Read the model definition and answer for the solid it produces. Units are mm, in the model's axes. A direction names the side the tool comes from. Coordinates: 2 decimals unless noted, no trailing zeros. Order: outer loops, then holes, each group sorted by start corner. A loop starts at its lowest first (then second) coordinate and runs counter-clockwise, first axis right, second up. Notation, with made-up numbers: (11.25, -29.5) -> (50.25, -29.5) arc R17 cw to (50.25, -22.5) -> close; hole circle Ø2 at (32, 68). An arc over 180 degrees is marked (long way). Answer in a Markdown table with one row per item.
from build123d import *

# Parameters (mm, degrees)
SKETCH1_W           = 35
SKETCH1_H           = 40
BOSS_EXTRUDE1_DEPTH = 2
SKETCH2_R           = 2.5
CUT_EXTRUDE1_DEPTH  = 54.188344588
SKETCH3_R           = 5.071067812
BOSS_EXTRUDE2_DEPTH = 35


with BuildPart() as part:
    # Sketch1 → Boss-Extrude1 (new body)
    with BuildSketch(Plane.XY):
        with Locations((17.5, 20)):
            Rectangle(SKETCH1_W, SKETCH1_H)
    extrude(amount=BOSS_EXTRUDE1_DEPTH)

    # Sketch2 → Cut-Extrude1 (cut, through all)
    with BuildSketch(Plane(origin=(0, 0, 0), x_dir=(-1, 0, 0), z_dir=(0, 0, -1))):
        with Locations((-27, 24)):
            Circle(SKETCH2_R)
        with Locations((-8, 24)):
            Circle(SKETCH2_R)
        with Locations((-8, 7.5)):
            Circle(SKETCH2_R)
        with Locations((-27, 7.5)):
            Circle(SKETCH2_R)
    extrude(amount=-CUT_EXTRUDE1_DEPTH, mode=Mode.SUBTRACT)

    # Sketch3 → Boss-Extrude2 (add)
    with BuildSketch(Plane.ZY):
        with BuildLine():
            Line((0, 40), (2, 40))
            Line((2, 40), (2, 44))
            ThreePointArc((2, 44), (1, 58.071067812), (0, 44))
            Line((0, 44), (0, 40))
        make_face()
        with Locations((1, 51)):
            Circle(SKETCH3_R, mode=Mode.SUBTRACT)
    extrude(amount=-BOSS_EXTRUDE2_DEPTH)


solid = part.part
Q1. The part is cut by section A-A (z = 1). Write down the section's boundary in (x, y).
Outcome:
| item | result |
|---|---|
| outline | (0, 0) -> (35, 0) -> (35, 45.93) -> (0, 45.93) -> close; (0, 56.07) -> (35, 56.07) -> (35, 58.07) -> (0, 58.07) -> close; hole circle Ø5 at (8, 7.5); hole circle Ø5 at (8, 24); hole circle Ø5 at (27, 7.5); hole circle Ø5 at (27, 24) |
Q2. The part is cut by section B-B (x = 27). Write down the section's boundary in (y, z), then the cut area to 3 significant figures.
Outcome:
| item | result |
|---|---|
| outline | (0, 0) -> (5, 0) -> (5, 2) -> (0, 2) -> close; (10, 0) -> (21.5, 0) -> (21.5, 2) -> (10, 2) -> close; (26.5, 0) -> (44, 0) arc R7.07 ccw (long way) to (44, 2) -> (26.5, 2) -> close; hole circle Ø10.14 at (51, 1) |
| area | 144 mm² |
Q3. For a pull along Z with two mould halves and no side action, classify faces 3 (the face through (17, 0, 1)), 4 (the face through (17.255, 56.028, 0.34)), 5 (the face through (17, 22, 2)) as pulls with the +Z half, pulls with the -Z half, needs draft (parallel to the pull), parting line crosses it, or undercut.
Outcome:
| item | result |
|---|---|
| face 3 | needs draft |
| face 4 | undercut |
| face 5 | pulls with the +Z half |
Q4. For faces 1 (the face through (28.84, 25.69, 0.99)), 2 (the face through (17, 22, 0)), determine the directions among +Z, -Z, +X, -X, +Y, -Y from which every point of the face is accessible in a straight line to the end or side of a thin tool.
Outcome:
| item | result |
|---|---|
| face 1 | +Z, -Z |
| face 2 | -Z, +X, -X, -Y |
Q5. The part is cut by section C-C (y = 7.5). Write down the section's boundary in (x, z).
Outcome:
| item | result |
|---|---|
| outline | (0, 0) -> (5.5, 0) -> (5.5, 2) -> (0, 2) -> close; (10.5, 0) -> (24.5, 0) -> (24.5, 2) -> (10.5, 2) -> close; (29.5, 0) -> (35, 0) -> (35, 2) -> (29.5, 2) -> close |
Q6. Consider line 1 (Y direction, x = 27, z = 1.25); line 2 (Y direction, x = 8, z = 0.5); line 3 (Z direction, x = 18.5, y = 13.5). Determine where each line is inside the solid, lowest interval first.
Outcome:
| item | result |
|---|---|
| line 1 | 0 to 5, 10 to 21.5, 26.5 to 45.94, 56.06 to 58.07 |
| line 2 | 0 to 5, 10 to 21.5, 26.5 to 45.95, 56.05 to 58.05 |
| line 3 | 0 to 2 |
Q7. The part is cut by section D-D (x = 22.5). Write down the section's boundary in (y, z), then the cut area to 3 significant figures.
Outcome:
| item | result |
|---|---|
| outline | (0, 0) -> (44, 0) arc R7.07 ccw (long way) to (44, 2) -> (0, 2) -> close; hole circle Ø10.14 at (51, 1) |
| area | 164 mm² |
Q8. Given pin 1 (10 mm diameter, centred on x = 11.5, y = 25, fed in from +Z); pin 2 (5 mm diameter, centred on y = 48, z = 4.5, fed in from -X); pin 3 (10 mm diameter, centred on x = 3.5, y = 41, fed in from -Z); pin 4 (3 mm diameter, centred on x = 27, y = 24, fed in from +Z), each flat-ended and moving along its own axis, determine where each tip first touches the part or whether it passes through.
Outcome:
| item | result |
|---|---|
| pin 1 | z = 2 |
| pin 2 | x = 0 |
| pin 3 | z = -4 |
| pin 4 | through |
